Verification items for the finished model (mm, model axes). Coordinates: 2 decimals unless noted, no trailing zeros. Write each loop counter-clockwise with the first axis right and the second up, starting at its lowest first coordinate (ties: lowest second). Pieces come first, ordered by that corner, then holes. Notation, with made-up numbers: (19.5, -24) -> (44.5, -24) arc R31 cw to (44.5, 13) -> close; hole circle Ø11 at (25, 12.25). An arc over 180 degrees is marked (long way). Write item = value, one per line. Start each with the question number.
(1) Section check A-A (z = 2). Record the cut outline in (x, y).
(2) Section check D-D (x = 9). Record the cut outline in (y, z), plus the area to 3 significant figures.
(3) Section check B-B (x = 5.25). Record the cut outline in (y, z).
(4) Mould release check, pull along X, two halves, no side actions. Record for faces 1 (the face through (-14, 1, 0)), 2 (the face through (14, 1, 0)), 3 (the face through (9.03, 0.99, -10.27)): released by +X, released by -X, zero draft, split by the parting line, or undercut.
(5) Material ranges on probe 1 along X at (y, z) = (0.85, -9); probe 2 along Z at (x, y) = (9, 1.8); probe 3 along X at (y, z) = (1.8, 0), recorded low to high. Write a range as [from, to].
(6) Section check C-C (y = 0.95). Record the cut outline in (x, z).
```python
from build123d import *

# Parameters (mm, degrees)
SKETCH_1_W          = 28
SKETCH_1_H          = 26
SKETCH_1_R          = 1.6
EXTRUDE_1_DEPTH     = 2
SKETCH_2_R          = 7.5
CUT_EXTRUDE_1_DEPTH = 2
FILLET_1_R          = 4


with BuildPart() as part:
    # 草图1 → 凸台-拉伸1 (new body)
    with BuildSketch(Plane(origin=(0, 0, 0), x_dir=(1, 0, 0), z_dir=(0, 1, 0))):
        Rectangle(SKETCH_1_W, SKETCH_1_H)
        with Locations(Location((10, -9, 0), (0, 0, 270))):
            Circle(SKETCH_1_R, mode=Mode.SUBTRACT)
        with Locations(Location((-10, -9, 0), (0, 0, 270))):
            Circle(SKETCH_1_R, mode=Mode.SUBTRACT)
        with Locations(Location((-10, 9, 0), (0, 0, 270))):
            Circle(SKETCH_1_R, mode=Mode.SUBTRACT)
        with Locations(Location((10, 9, 0), (0, 0, 270))):
            Circle(SKETCH_1_R, mode=Mode.SUBTRACT)
    extrude(amount=EXTRUDE_1_DEPTH)

    # 草图2 → 切除-拉伸1 (cut)
    with BuildSketch(Plane(origin=(0, 2, 0), x_dir=(1, 0, 0), z_dir=(0, 1, 0))):
        with Locations(Location((0, 0, 0), (0, 0, 270))):
            Circle(SKETCH_2_R)
    extrude(amount=-CUT_EXTRUDE_1_DEPTH, mode=Mode.SUBTRACT)

    # 圆角1
    fillet_1_edges = [part.edges().sort_by_distance(p)[0] for p in [
        (14, 1, 13),
        (-14, 1, 13),
        (-14, 1, -13),
        (14, 1, -13),
    ]]
    fillet(fillet_1_edges, radius=FILLET_1_R)


solid = part.part
```
Response:
q1.outline = (-14, 0) -> (-7.23, 0) -> (-7.23, 2) -> (-14, 2) -> close; (7.23, 0) -> (14, 0) -> (14, 2) -> (7.23, 2) -> close
q2.outline = (0, -13) -> (2, -13) -> (2, -10.25) -> (0, -10.25) -> close; (0, -7.75) -> (2, -7.75) -> (2, 7.75) -> (0, 7.75) -> close; (0, 10.25) -> (2, 10.25) -> (2, 13) -> (0, 13) -> close
q2.area = 42.0 mm2
q3.outline = (0, -13) -> (2, -13) -> (2, -5.36) -> (0, -5.36) -> close; (0, 5.36) -> (2, 5.36) -> (2, 13) -> (0, 13) -> close
q4.face_1 = released by -X
q4.face_2 = released by +X
q4.face_3 = undercut
q5.probe_1 = [-14, -11.6], [-8.4, 8.4], [11.6, 14]
q5.probe_2 = [-13, -10.25], [-7.75, 7.75], [10.25, 13]
q5.probe_3 = [-14, -7.5], [7.5, 14]
q6.outline = (-14, -9) arc R4 ccw to (-10, -13) -> (10, -13) arc R4 ccw to (14, -9) -> (14, 9) arc R4 ccw to (10, 13) -> (-10, 13) arc R4 ccw to (-14, 9) -> close; hole circle Ø3.2 at (-10, -9); hole circle Ø3.2 at (-10, 9); hole circle Ø15 at (0, 0); hole circle Ø3.2 at (10, -9); hole circle Ø3.2 at (10, 9)
